from build123d import *

# Parameters (mm, degrees)
F0_R     = 2
F1_DEPTH = 0.4


# Not quite as in the source:
# - a pattern or mirror of a feature is missing from the dataset's text; its kind, count and spacing are read off the source's solid


with BuildPart() as f1:
    # F0 (on Top) → F1 (new body)
    with BuildSketch(Plane.XY):
        with BuildLine():
            Line((-8, -34.5), (8, -34.5))
            ThreePointArc((8, -34.5), (9.4142135624, -33.9142135624), (10, -32.5))
            Line((10, -32.5), (10, 34.5))
            ThreePointArc((10, 34.5), (7, 37.5), (4, 34.5))
            Line((4, 34.5), (4, 24.8))
            Line((4, 24.8), (-4, 24.8))
            Line((-4, 24.8), (-4, 34.5))
            ThreePointArc((-4, 34.5), (-7, 37.5), (-10, 34.5))
            Line((-10, 34.5), (-10, -32.5))
            ThreePointArc((-10, -32.5), (-9.4142135624, -33.9142135624), (-8, -34.5))
        make_face()
        with BuildLine():
            Line((-7, -28), (-7, 0))
            Line((-7, 0), (-5, 0))
            Line((-5, 0), (5, 0))
            Line((5, 0), (7, 0))
            Line((7, 0), (7, -28))
            ThreePointArc((7, -28), (6.4142135624, -29.4142135624), (5, -30))
            Line((5, -30), (-5, -30))
            ThreePointArc((-5, -30), (-6.4142135624, -29.4142135624), (-7, -28))
        make_face(mode=Mode.SUBTRACT)
        with Locations((-5, 19.5)):
            Circle(F0_R, mode=Mode.SUBTRACT)
        with BuildLine():
            ThreePointArc((-5, 14.8603921946), (0, 11.5), (5, 14.8603921946))
            ThreePointArc((5, 14.8603921946), (6.3036310751, 15.4086129713), (6.8518518519, 14.1049818963))
            ThreePointArc((6.8518518519, 14.1049818963), (0, 9.5), (-6.8518518519, 14.1049818963))
            ThreePointArc((-6.8518518519, 14.1049818963), (-6.3036310751, 15.4086129713), (-5, 14.8603921946))
        make_face(mode=Mode.SUBTRACT)
        with Locations((5, 19.5)):
            Circle(F0_R, mode=Mode.SUBTRACT)
        with BuildLine():
            Line((5, 0), (-5, 0))
            Line((-5, 0), (-5, -17))
            ThreePointArc((-5, -17), (0, -22), (5, -17))
            Line((5, -17), (5, 0))
        make_face()
    extrude(amount=F1_DEPTH)

    # F1_copies: F1 across plane


with BuildPart() as f1_1:
    add(f1.part)
    add(f1.part.mirror(Plane.XY.offset(0.3)))


solid = f1_1.part
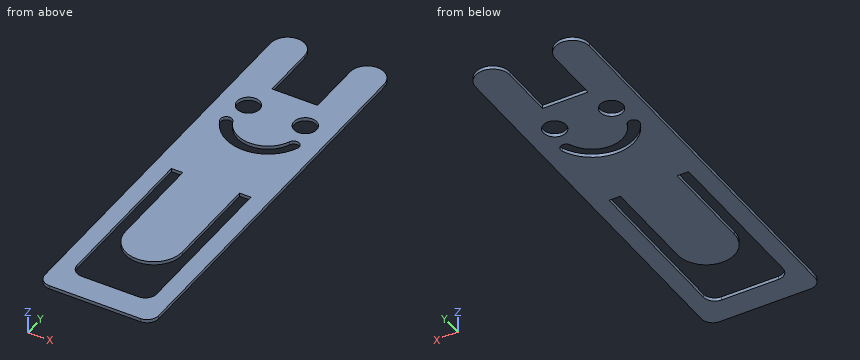
Verification items for the finished model (mm, model axes). Coordinates: 2 decimals unless noted, no trailing zeros. Write each loop counter-clockwise with the first axis right and the second up, starting at its lowest first coordinate (ties: lowest second). Pieces come first, ordered by that corner, then holes. Notation, with made-up numbers: (-23, 3.25) -> (33, 3.25) arc R22 ccw to (33, 30.25) -> close; hole circle Ø11 at (84.25, 30). An arc over 180 degrees is marked (long way). One line per item, written item: value. Start each with the question number.
Q1. Cross-section at B-B on x = 0. Enter the section's corners in (y, z), and give its area (3 significant figures).
Q2. Thickness scan on L1, parallel to X at y = -15.5, z = 0.2; L2, parallel to Y at x = -2.25, z = 0.4; L3, parallel to Y at x = -4.5, z = 0.5. Record the ranges inside material, lowest first. Write a range as from..to.
Q3. Go/stop test with a flat-tipped pin: P1, Ø5, axis at x = -5, y = 19.5, coming from the +Z side. Record where the tip stops, or that it passes through.
Q4. Cross-section at A-A on z = 0.1. Enter the section's corners in (x, y), and give its area (3 significant figures).
Q5. Cross-section at C-C on y = 31.5. Enter the section's corners in (x, z).
Checked values:
1. outline: (-34.5, 0) -> (-30, 0) -> (-30, 0.6) -> (-34.5, 0.6) -> close; (-22, 0) -> (9.5, 0) -> (9.5, 0.6) -> (-22, 0.6) -> close; (11.5, 0) -> (24.8, 0) -> (24.8, 0.6) -> (11.5, 0.6) -> close
1. area: 29.6 mm²
2. L1: x = -10..-7, -5..5, 7..10
2. L2: y = -34.5..-30, -21.47..9.85, 11.99..24.8
2. L3: y = -34.5..-30, -19.18..11.03, 13.92..17.56, 21.44..36.16
3. P1: stops at z = 0.6
4. outline: (-10, -32.5) arc R2 ccw to (-8, -34.5) -> (8, -34.5) arc R2 ccw to (10, -32.5) -> (10, 34.5) arc R3 ccw to (4, 34.5) -> (4, 24.8) -> (-4, 24.8) -> (-4, 34.5) arc R3 ccw to (-10, 34.5) -> close; hole (-7, -28) arc R2 ccw to (-5, -30) -> (5, -30) arc R2 ccw to (7, -28) -> (7, 0) -> (5, 0) -> (5, -17) arc R5 cw to (-5, -17) -> (-5, 0) -> (-7, 0) -> close; hole circle Ø4 at (-5, 19.5); hole (-6.85, 14.1) arc R7.4 ccw to (6.85, 14.1) arc R1 ccw to (5, 14.86) arc R5.4 cw to (-5, 14.86) arc R1 ccw to start; hole circle Ø4 at (5, 19.5)
4. area: 1,060 mm²
5. outline: (-10, 0) -> (-4, 0) -> (-4, 0.6) -> (-10, 0.6) -> close; (4, 0) -> (10, 0) -> (10, 0.6) -> (4, 0.6) -> close
